Read the model definition and answer for the solid it produces. Units are mm, in the model's axes. Give positions to 0.01 mm unless a question says otherwise; leave off trailing zeros. Write each loop counter-clockwise with the first axis right and the second up, starting at its lowest first coordinate (ties: lowest second). Pieces come first, ordered by that corner, then holes. Notation, with made-up numbers: (-7.5, 17) -> (5.5, 17) arc R22 ccw to (5.5, 53) -> close; hole circle Ø3 at (-10.75, -3.75). An arc over 180 degrees is marked (long way). Write item = value, one per line.
from build123d import *

# Parameters (mm, degrees)
SKETCH089_W             = 27
SKETCH089_H             = 27
SKETCH089_R             = 1.5
PAD036_DEPTH            = 3
SKETCH088_R             = 11.5
SKETCH088_R_2           = 1.6
PAD037_DEPTH            = 3
PAD038_DEPTH            = 27
SKETCH092_W             = 3
SKETCH092_H             = 29.5
PAD039_DEPTH            = 10.9
SKETCH093_W             = 3
SKETCH093_H             = 29.5
PAD040_DEPTH            = 70.9
PAD040_DEPTH_BACK       = 3
SKETCH094_W             = 3
SKETCH094_H             = 4
PAD041_DEPTH            = 73.9
SKETCH095_W             = 1
SKETCH095_H             = 3
SKETCH095_W_2           = 2
SKETCH095_H_2           = 2
POCKET048_DEPTH         = 74
SKETCH096_R             = 1
POCKET049_DEPTH         = 3
PAD042_DEPTH            = 29.5
BODY010_ROLL_ANGLE      = -89.9826768737
BODY010_PITCH_ANGLE     = -0.0173178896
BODY010_PLACEMENT_ANGLE = 89.9826768737


with BuildPart() as part:
    # Sketch089 → Pad036 (new body)
    with BuildSketch(Plane.XZ):
        with Locations((13.5, -13.5)):
            Rectangle(SKETCH089_W, SKETCH089_H)
        with Locations((7, -16.5)):
            Circle(SKETCH089_R, mode=Mode.SUBTRACT)
        with Locations((13.5, -19.5)):
            Circle(SKETCH089_R, mode=Mode.SUBTRACT)
        with Locations((20, -16.5)):
            Circle(SKETCH089_R, mode=Mode.SUBTRACT)
    extrude(amount=-PAD036_DEPTH)

    # Sketch088 → Pad037 (join)
    with BuildSketch(Plane.XY):
        with BuildLine():
            Line((0, 42), (0, 0))
            Line((0, 0), (27, 0))
            Line((27, 0), (27, 42))
            ThreePointArc((27, 42), (26.1213203436, 44.1213203436), (24, 45))
            Line((24, 45), (3, 45))
            ThreePointArc((3, 45), (0.8786796564, 44.1213203436), (0, 42))
        make_face()
        with Locations((13.5, 29.5)):
            Circle(SKETCH088_R, mode=Mode.SUBTRACT)
        with Locations((3.8, 39.2)):
            Circle(SKETCH088_R_2, mode=Mode.SUBTRACT)
        with Locations((23.2, 39.2)):
            Circle(SKETCH088_R_2, mode=Mode.SUBTRACT)
        with Locations((23.2, 19.8)):
            Circle(SKETCH088_R_2, mode=Mode.SUBTRACT)
        with Locations((3.8, 19.8)):
            Circle(SKETCH088_R_2, mode=Mode.SUBTRACT)
    extrude(amount=PAD037_DEPTH)

    # Sketch090 → Pad038 (join)
    with BuildSketch(Plane.YZ):
        with BuildLine():
            ThreePointArc((10, 0), (2.9289309634, -2.9289334129), (0, -10.0000034641))
            Line((0, -10.000003), (0, 0))
            Line((10, 0), (0, 0))
        make_face()
    extrude(amount=PAD038_DEPTH)

    # Sketch092 (on Face17 of Pad038) → Pad039 (join)
    with BuildSketch(Plane(origin=(0, 0, 0), x_dir=(0, 0, -1), z_dir=(-1, 0, 0))):
        with Locations((-1.5, -14.75)):
            Rectangle(SKETCH092_W, SKETCH092_H)
    extrude(amount=PAD039_DEPTH)

    # Sketch093 (on Face21 of Pad039) → Pad040 (join, two sides)
    with BuildSketch(Plane(origin=(0, 0, 3), x_dir=(-1, 0, 0), z_dir=(0, 0, 1))) as pad040_sk:
        with Locations((12.4, -14.75)):
            Rectangle(SKETCH093_W, SKETCH093_H)
    extrude(amount=PAD040_DEPTH)
    extrude(pad040_sk.sketch, amount=-PAD040_DEPTH_BACK)

    # Sketch094 (on Face20 of Pad040) → Pad041 (join)
    with BuildSketch(Plane(origin=(0, 0, 73.9), x_dir=(-1, 0, 0), z_dir=(0, 0, 1))):
        with Locations((15.4, -11)):
            Rectangle(SKETCH094_W, SKETCH094_H)
        with Locations((15.4, -18.5)):
            Rectangle(SKETCH094_W, SKETCH094_H)
    extrude(amount=-PAD041_DEPTH)

    # Sketch095 (on Face32 of Pad041) → Pocket048 (cut)
    with BuildSketch(Plane(origin=(0, 0, 73.9), x_dir=(-1, 0, 0), z_dir=(0, 0, 1))):
        with Locations((14.4, -11)):
            Rectangle(SKETCH095_W, SKETCH095_H)
        with Locations((15.9, -11)):
            Rectangle(SKETCH095_W_2, SKETCH095_H_2)
        with Locations((14.4, -18.5)):
            Rectangle(SKETCH095_W, SKETCH095_H)
        with Locations((15.9, -18.5)):
            Rectangle(SKETCH095_W_2, SKETCH095_H_2)
    extrude(amount=-POCKET048_DEPTH, mode=Mode.SUBTRACT)

    # Sketch096 (on Face20 of Pocket048) → Pocket049 (cut)
    with BuildSketch(Plane(origin=(-13.9, 0, 0), x_dir=(0, 0, -1), z_dir=(-1, 0, 0))):
        with Locations((-10, -14.7)):
            Circle(SKETCH096_R)
    extrude(amount=-POCKET049_DEPTH, mode=Mode.SUBTRACT)

    # Sketch097 (on Face33 of Pocket049) → Pad042 (join)
    with BuildSketch(Plane.XZ):
        with BuildLine():
            ThreePointArc((-11.1945579857, 6.3643060843), (-9.8282285955, 4.1860605156), (-7.686876766, 2.76260623))
            Line((-7.686877, 2.762606), (-11.55202, 1.663341))
            Line((-11.194558, 6.364306), (-11.55202, 1.663341))
        make_face()
    extrude(amount=-PAD042_DEPTH)


with BuildPart() as part_1:
    # Body010 roll: moved
    add(part.part.rotate(Axis((0, 0, 0), (1, 0, 0)), BODY010_ROLL_ANGLE))


with BuildPart() as part_2:
    # Body010 pitch: moved
    add(part_1.part.rotate(Axis((0, 0, 0), (0, 1, 0)), BODY010_PITCH_ANGLE))


with BuildPart() as part_3:
    # Body010 placement: moved
    add(part_2.part.moved(Location((-70, 7, 0))).rotate(Axis((-70, 7, 0), (0, 0, 1)), BODY010_PLACEMENT_ANGLE))


solid = part_3.part
(1) Given P1, Ø8, axis at y = 12, z = -35.5, coming from the +X side; P2, Ø4, axis at x = -65, y = 4, coming from the +Z side; P3, Ø0.8, axis at x = -120.5, y = -7.5, coming from the -Z side; P4, Ø2, axis at x = -113, y = -8.5, coming from the +Z side, each flat-ended and moving along its own axis, determine where each tip first touches the part or whether it passes through.
Checks:
P1 = -70.01
P2 = through
P3 = -20.49
P4 = -8.99
(2) The part is cut by section B-B on y = 27.5. Count the separate pieces of the cut face and the enclosed holes in it, plus the area to 3 significant figures.
Checks:
separate_pieces = 3
enclosed_holes = 0
area = 159 mm²
(3) Consider L1, parallel to Z at x = -107, y = -7; L2, parallel to Z at x = -49, y = 30; L3, parallel to X at y = 7, z = -21.5. Determine where each line is inside the solid, lowest interval first.
Checks:
L1 = -20.49 to -19.99, -16.99 to -16.49, -12.99 to -12.49, -9.49 to -8.99
L2 = -3 to 0
L3 = -73.01 to -70.01
(4) The part is cut by section A-A on x = -112. Determine the outline of the cut face in (y, z).
Checks:
outline = (-9.88, -20.49) -> (-6.88, -20.49) -> (-6.88, -29.49) -> (-3.88, -29.49) -> (-3.89, 0.01) -> (-6.89, 0.01) -> (-6.88, -8.99) -> (-9.88, -8.99) -> (-9.88, -9.99) -> (-7.88, -9.99) -> (-7.88, -9.49) -> (-6.88, -9.49) -> (-6.88, -12.49) -> (-7.88, -12.49) -> (-7.88, -11.99) -> (-9.88, -11.99) -> (-9.88, -12.99) -> (-6.88, -12.99) -> (-6.88, -16.49) -> (-9.88, -16.49) -> (-9.88, -17.49) -> (-7.88, -17.49) -> (-7.88, -16.99) -> (-6.88, -16.99) -> (-6.88, -19.99) -> (-7.88, -19.99) -> (-7.88, -19.49) -> (-9.88, -19.49) -> close
(5) For a pull along Z with two mould halves and no side action, classify faces 1 (the cylindrical face through (-71.48, 30.94, -18.37)), 2 (the cylindrical face through (-54.98, 26.8, -1.48)) as released by +Z, released by -Z, zero draft, split by the parting line, or undercut.
Checks:
face_1 = undercut
face_2 = split by the parting line
